The listing builds one solid part. Answer for the finished solid, in the listing's coordinates (mm). A direction names the side the tool comes from. Give positions to 0.01 mm unless a question says otherwise; leave off trailing zeros. Write each loop counter-clockwise with the first axis right and the second up, starting at its lowest first coordinate (ties: lowest second). Pieces come first, ordered by that corner, then holes.
```python
from build123d import *

# Parameters (mm, degrees)
SKETCH_1_R           = 18.5
SKETCH_1_R_2         = 18
EXTRUDE_1_DEPTH      = 180
CUT_EXTRUDE_1_DEPTH  = 30
SKETCH_5_R           = 1.5
EXTRUDE_2_DEPTH      = 5
SKETCH_8_R           = 1.5
CUT_EXTRUDE_2_DEPTH  = 2
SKETCH_9_R           = 1.5
CUT_EXTRUDE_3_DEPTH  = 2
SKETCH_12_W          = 21.543450216
SKETCH_12_H          = 50.101047014
CUT_EXTRUDE_4_DEPTH  = 201
SKETCH_13_W          = 20
SKETCH_13_H          = 0.5
EXTRUDE_3_DEPTH      = 40
SKETCH_14_W          = 20
SKETCH_14_H          = 1
CUT_EXTRUDE_5_DEPTH  = 40
EXTRUDE_4_DEPTH      = 0.5
CUT_EXTRUDE_25_DEPTH = 0.5
CUT_EXTRUDE_26_DEPTH = 0.5
CUT_EXTRUDE_27_DEPTH = 0.5


with BuildPart() as part:
    # 草图1 → 凸台-拉伸1 (new body)
    with BuildSketch(Plane.XY):
        with Locations(Location((0, 0, 0), (0, 0, 180))):
            Circle(SKETCH_1_R)
        with Locations(Location((0, 0, 0), (0, 0, 180))):
            Circle(SKETCH_1_R_2, mode=Mode.SUBTRACT)
    extrude(amount=EXTRUDE_1_DEPTH)

    # 草图4 → 切除-拉伸1 (cut, symmetric)
    with BuildSketch(Plane(origin=(0, 0, 0), x_dir=(0, 0, -1), z_dir=(1, 0, 0))):
        with BuildLine():
            Line((-2.121320344, -16.378679656), (-8.485281374, -10.014718626))
            ThreePointArc((-8.485281374, -10.014718626), (-4.592201188, -7.41344561), (0, -6.5))
            Line((0, -6.5), (0, -15.5))
            ThreePointArc((0, -15.5), (-1.148050297, -15.728361402), (-2.121320344, -16.378679656))
        make_face()
        with BuildLine():
            Line((-23.744748589, 23.215547635), (0, 23.215547635))
            Line((0, 23.215547635), (0, 20.5))
            ThreePointArc((0, 20.5), (-14.924653862, 17.531301768), (-27.577164466, 9.077164466))
            Line((-27.577164466, 9.077164466), (-33.941125497, 15.441125497))
            ThreePointArc((-33.941125497, 15.441125497), (-29.103701262, 19.670336295), (-23.744748589, 23.215547635))
        make_face()
        with BuildLine():
            Line((-14.849242405, -3.650757595), (-21.213203436, 2.713203436))
            ThreePointArc((-21.213203436, 2.713203436), (-11.480502971, 9.216385975), (0, 11.5))
            Line((0, 11.5), (0, 2.5))
            ThreePointArc((0, 2.5), (-8.03635208, 0.901470183), (-14.849242405, -3.650757595))
        make_face()
    extrude(amount=CUT_EXTRUDE_1_DEPTH, both=True, mode=Mode.SUBTRACT)

    # 草图5 → 凸台-拉伸2 (add, symmetric)
    with BuildSketch(Plane(origin=(0, 0, 0), x_dir=(0, 0, -1), z_dir=(1, 0, 0))):
        with BuildLine():
            Line((-0.190075543, -18), (-2.072124505, -18))
            ThreePointArc((-2.072124505, -18), (1.060660172, -23.060660172), (4.193444848, -18))
            Line((4.193444848, -18), (2.311395887, -18))
            ThreePointArc((2.311395887, -18), (1.060660172, -17.560660172), (-0.190075543, -18))
        make_face()
        with Locations((1.060660172, -19.560660172)):
            Circle(SKETCH_5_R, mode=Mode.SUBTRACT)
    extrude(amount=EXTRUDE_2_DEPTH, both=True)

    # 草图8 → 切除-拉伸2 (cut)
    with BuildSketch(Plane(origin=(3.5, 0, 0), x_dir=(0, 0, -1), z_dir=(1, 0, 0))):
        with BuildLine():
            Line((-0.190075543, -18), (-2.072124505, -18))
            ThreePointArc((-2.072124505, -18), (1.060660172, -23.060660172), (4.193444848, -18))
            Line((4.193444848, -18), (2.311395887, -18))
            ThreePointArc((2.311395887, -18), (1.060660172, -17.560660172), (-0.190075543, -18))
        make_face()
        with Locations((1.060660172, -19.560660172)):
            Circle(SKETCH_8_R, mode=Mode.SUBTRACT)
    extrude(amount=-CUT_EXTRUDE_2_DEPTH, mode=Mode.SUBTRACT)

    # 草图9 → 切除-拉伸3 (cut)
    with BuildSketch(Plane(origin=(-1.5, 0, 0), x_dir=(0, 0, -1), z_dir=(1, 0, 0))):
        with BuildLine():
            Line((-2.072124505, -18), (-0.190075543, -18))
            ThreePointArc((-0.190075543, -18), (1.060660172, -17.560660172), (2.311395887, -18))
            Line((2.311395887, -18), (4.193444848, -18))
            ThreePointArc((4.193444848, -18), (1.060660172, -23.060660172), (-2.072124505, -18))
        make_face()
        with Locations((1.060660172, -19.560660172)):
            Circle(SKETCH_9_R, mode=Mode.SUBTRACT)
    extrude(amount=-CUT_EXTRUDE_3_DEPTH, mode=Mode.SUBTRACT)

    # 草图12 → 切除-拉伸4 (cut, symmetric)
    with BuildSketch(Plane(origin=(0, 0, 0), x_dir=(-1, 0, 0), z_dir=(0, 0, -1))):
        with Locations((-10.771725108, -0.713406874)):
            Rectangle(SKETCH_12_W, SKETCH_12_H)
    extrude(amount=CUT_EXTRUDE_4_DEPTH, both=True, mode=Mode.SUBTRACT)

    # 草图13 → 凸台-拉伸3 (add)
    with BuildSketch(Plane(origin=(0, 0, 0), x_dir=(0, 0, -1), z_dir=(1, 0, 0))):
        with Locations((-110, -18.25)):
            Rectangle(SKETCH_13_W, SKETCH_13_H)
        with Locations((-70, -18.25)):
            Rectangle(SKETCH_13_W, SKETCH_13_H)
        with Locations((-150, -18.25)):
            Rectangle(SKETCH_13_W, SKETCH_13_H)
    extrude(amount=EXTRUDE_3_DEPTH)

    # 草图14 → 切除-拉伸5 (cut)
    with BuildSketch(Plane(origin=(0, 0, 0), x_dir=(0, 0, -1), z_dir=(1, 0, 0))):
        with Locations((-90, -18)):
            Rectangle(SKETCH_14_W, SKETCH_14_H)
        with Locations((-50, -18)):
            Rectangle(SKETCH_14_W, SKETCH_14_H)
        with Locations((-130, -18)):
            Rectangle(SKETCH_14_W, SKETCH_14_H)
        with Locations((-170, -18)):
            Rectangle(SKETCH_14_W, SKETCH_14_H)
    extrude(amount=-CUT_EXTRUDE_5_DEPTH, mode=Mode.SUBTRACT)

    # 草图16 → 凸台-拉伸4 (add)
    with BuildSketch(Plane.XZ.offset(18.5)):
        with BuildLine():
            Line((39.998675576, 44.557290849), (39.998953647, 68.795192772))
            ThreePointArc((39.998953647, 68.795192772), (20.682117379, 76.824270149), (0, 79.963739473))
            Line((0, 79.963739473), (0, 59.952777719))
            ThreePointArc((0, 59.952777719), (21.279727814, 55.581587428), (39.998675576, 44.557290849))
        make_face()
        with BuildLine():
            Line((0, 11.92), (0, 39.932309719))
            ThreePointArc((0, 39.932309719), (24.002531018, 31.642513786), (39.998301143, 11.92))
            Line((39.998301143, 11.92), (0, 11.92))
        make_face()
        with BuildLine():
            Line((0, 159.981196289), (0, 139.978623608))
            ThreePointArc((0, 139.978623608), (20.218739097, 138.224024642), (39.999698116, 133.686438442))
            Line((39.999698116, 133.686438442), (39.999936605, 154.474190176))
            ThreePointArc((39.999936605, 154.474190176), (20.167826378, 158.446924196), (0, 159.981196289))
        make_face()
        with BuildLine():
            Line((39.999209833, 91.125521645), (39.999456529, 112.628600071))
            ThreePointArc((39.999456529, 112.628600071), (20.297610274, 117.92376471), (0, 119.975235288))
            Line((0, 119.975235288), (0, 99.97057031))
            ThreePointArc((0, 99.97057031), (20.430131767, 97.494980868), (39.999209833, 91.125521645))
        make_face()
    extrude(amount=-EXTRUDE_4_DEPTH)

    # 草图20 → 切除-拉伸25 (cut)
    with BuildSketch(Plane.XZ.offset(18.5)):
        with BuildLine():
            Line((40, 80), (40, 68.794599806))
            ThreePointArc((40, 68.794599806), (20.682696569, 76.824108425), (0, 79.963739473))
            Line((0, 79.963739473), (0, 80))
            Line((0, 80), (40, 80))
        make_face()
    extrude(amount=-CUT_EXTRUDE_25_DEPTH, mode=Mode.SUBTRACT)

    # 草图22 → 切除-拉伸26 (cut)
    with BuildSketch(Plane.XZ.offset(18.5)):
        with BuildLine():
            Line((40, 120), (40, 112.628405695))
            ThreePointArc((40, 112.628405695), (20.297894119, 117.923712576), (0, 119.975235288))
            Line((0, 119.975235288), (0, 120))
            Line((0, 120), (40, 120))
        make_face()
    extrude(amount=-CUT_EXTRUDE_26_DEPTH, mode=Mode.SUBTRACT)

    # 草图23 → 切除-拉伸27 (cut)
    with BuildSketch(Plane.XZ.offset(18.5)):
        with BuildLine():
            Line((40, 160), (40, 154.474173407))
            ThreePointArc((40, 154.474173407), (20.167858859, 158.446919724), (0, 159.981196289))
            Line((0, 159.981196289), (0, 160))
            Line((0, 160), (40, 160))
        make_face()
    extrude(amount=-CUT_EXTRUDE_27_DEPTH, mode=Mode.SUBTRACT)


solid = part.part
```
Item 1: A cutting plane is placed at D-D, the plane y = -12.5. Give the vertices of the cut face in (x, z).
Conclusion:
outline: (-13.64, 6) - (-12.95, 6) - (-12.95, 180) - (-13.64, 180) - close
Item 2: Each of these flat-tipped pins is pushed along its axis until it touches: P1, Ø2, axis at y = -8, z = 132.5, coming from the -X side; P2, Ø1.2, axis at x = -6.5, y = -17, coming from the -Z side; P3, Ø3, axis at y = -5, z = 31.5, coming from the +X side. Where does it stop, or does it pass through?
Conclusion:
P1: stops at x = -17.12
P2: stops at z = 0
P3: stops at x = -16.79
Item 3: A cutting plane is placed at A-A, the plane x = 19. Give the vertices of the cut face in (y, z).
Conclusion:
outline: (-18.5, 11.92) - (-18, 11.92) - (-18, 34.69) - (-18.5, 34.69) - close; (-18.5, 56.41) - (-18, 56.41) - (-18, 77.28) - (-18.5, 77.28) - close; (-18.5, 97.8) - (-18, 97.8) - (-18, 118.16) - (-18.5, 118.16) - close; (-18.5, 138.41) - (-18, 138.41) - (-18, 158.6) - (-18.5, 158.6) - close
Item 4: Which of the six approach directions +Z, -Z, +X, -X, +Y, -Y give full straight-line access (tool end or side, diameter ignored) to faces 1 (the face through (16, -18, 23)), 2 (the face through (-7.7, 16.5, 0)), 3 (the face through (-18.154, 0.945, 7.93))?
Conclusion:
face 1: +Z, -Z, +X, +Y
face 2: -Z, +X, -X, +Y
face 3: +X, -X, +Y
Item 5: A cutting plane is placed at B-B, the plane y = 0. Give the vertices of the cut face in (x, z), plus the area to 3 significant figures.
Conclusion:
outline: (-18.5, 0) - (-18, 0) - (-18, 9.94) - (-18.5, 9.94) - close; (-18.5, 18.5) - (-18, 18.5) - (-18, 180) - (-18.5, 180) - close
area: 85.7 mm2
Item 6: Determine the mould class of faces 4 (the face through (20, -18, 106)), 5 (the face through (20.965, -18.254, 76.745)), 6 (the face through (-13.2, 12.5, 31)), 7 (the face through (-15.733, 9.195, 11.531)) for opening direction Z: pulls with the +Z half, pulls with the -Z half, needs draft (parallel to the pull), parting line crosses it, or undercut.
Conclusion:
face 4: needs draft
face 5: undercut
face 6: undercut
face 7: pulls with the -Z half
Item 7: A cutting plane is placed at C-C, the plane x = 35. Give the vertices of the cut face in (y, z) (3 decimals).
Conclusion:
outline: (-18.5, 11.92) - (-18, 11.92) - (-18, 20.785) - (-18.5, 20.785) - close; (-18.5, 48.354) - (-18, 48.354) - (-18, 71.416) - (-18.5, 71.416) - close; (-18.5, 93.159) - (-18, 93.159) - (-18, 114.3) - (-18.5, 114.3) - close; (-18.5, 135.109) - (-18, 135.109) - (-18, 155.714) - (-18.5, 155.714) - close
Item 8: Consider probe 1 along Y at (x, z) = (-1, 153.5); probe 2 along Y at (x, z) = (4, 29.5); probe 3 along X at (y, z) = (-0.5, 102). Determine where each line is inside the solid, lowest interval first.
Conclusion:
probe 1: y = -18.47 to -17.97, 17.97 to 18.47
probe 2: y = -18.5 to -18
probe 3: x = -18.49 to -17.99
